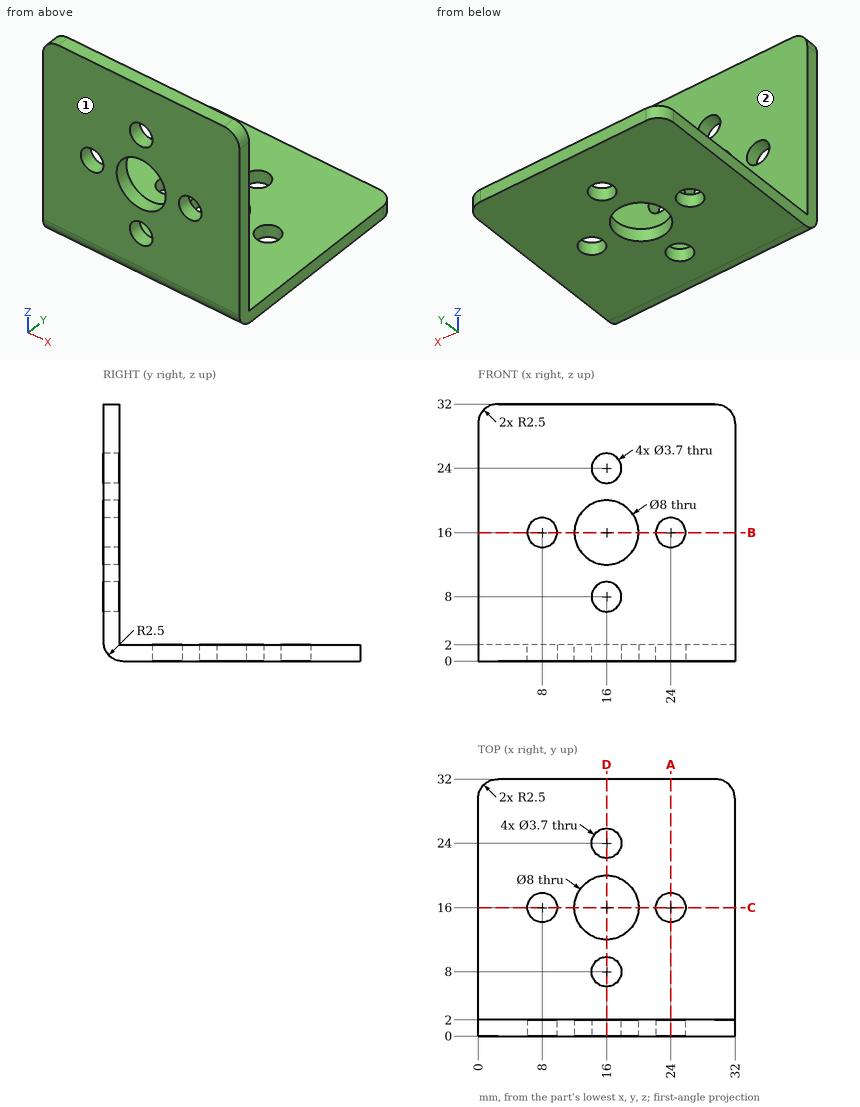
Print and shaded views of the part. All mm, measured from the part's lowest x, y and z. A direction names the side the tool comes from. Round coordinates to 2 decimals unless told otherwise and drop trailing zeros. Write each loop counter-clockwise with the first axis right and the second up, starting at its lowest first coordinate (ties: lowest second). Pieces come first, ordered by that corner, then holes. Notation, with made-up numbers: M 77,40.25 L 107,40.25 A19 cw 107,49.25 Z; hole C 38,36.25 d4. An arc over 180 degrees is marked long. Use a Markdown table: item, result. Add a question column.
1. Slice it at A-A on x = 24. Give the cut face in (y, z), then the cut area to 3 significant figures.
2. 3-axis set-ups, long thin cutter, end or side, ignore diameter. For the marked faces 1 and 2: which of +Z, -Z, +X, -X, +Y, -Y reach the whole face in a straight line?
3. Drill centre lines: probe 1 along Y at (x, z) = (16, 1); probe 2 along Z at (x, y) = (16, 1.15); probe 3 along Y at (x, z) = (28.5, 23). Where is each one in solid material? Low to high.
4. Slice it at B-B on z = 16. Give the cut face in (x, y).
5. Slice it at D-D on x = 16. Give the number of separate pieces and of enclosed holes in the cut face, then the cut area to 3 significant figures.
6. Flat gauge pins, fed straight in: P1, Ø9, axis at x = 16, y = 16, coming from the +Z side; P2, Ø4, axis at x = 8, z = 27, coming from the -Y side; P3, Ø7, axis at x = 16, z = 16, coming from the +Y side; P4, Ø15, axis at x = 13, z = 10, coming from the +Y side. Where does each tip first touch, or does it go through?
Reply:
| question | item | result |
|---|---|---|
| 1 | outline | M 0,2.5 A2.5 ccw 2.5,0 L 14.15,0 L 14.15,2 L 2,2 L 2,14.15 L 0,14.15 Z; M 0,17.85 L 2,17.85 L 2,32 L 0,32 Z; M 17.85,0 L 32,0 L 32,2 L 17.85,2 Z |
| 1 | area | 108 mm^2 |
| 2 | face 1 | +Z, -Z, +X, -X, -Y |
| 2 | face 2 | +Z, +X, -X, +Y |
| 3 | probe 1 | y = 0.5 to 6.15, 9.85 to 12, 20 to 22.15, 25.85 to 32 |
| 3 | probe 2 | z = 0.4 to 6.15, 9.85 to 12, 20 to 22.15, 25.85 to 32 |
| 3 | probe 3 | y = 0 to 2 |
| 4 | outline | M 0,0 L 6.15,0 L 6.15,2 L 0,2 Z; M 9.85,0 L 12,0 L 12,2 L 9.85,2 Z; M 20,0 L 22.15,0 L 22.15,2 L 20,2 Z; M 25.85,0 L 32,0 L 32,2 L 25.85,2 Z |
| 5 | separate pieces | 7 |
| 5 | enclosed holes | 0 |
| 5 | area | 61.1 mm^2 |
| 6 | P1 | stops at z = 2 |
| 6 | P2 | stops at y = 0 |
| 6 | P3 | passes through |
| 6 | P4 | stops at y = 2 |
